Part print with two shaded views. Sizes in mm from the minimum x, y, z corner. A direction names the side the tool comes from. Give positions to 0.01 mm unless a question says otherwise; leave off trailing zeros. Loops run counter-clockwise (first coordinate to the right, second up) from the corner with the lowest first, then second, coordinate; pieces in that order, holes last. Notation, with made-up numbers: (-14, 10) -> (34, 10) arc R23 ccw to (34, 26) -> close; hole circle Ø10 at (36.5, 7). An arc over 180 degrees is marked (long way). One line per question, with ' | ' between items. Start each with the question number.
(1) Slice it at B-B, the plane x = 35.5. Write the cut outline in (y, z).
(2) Drill centre lines: L1, parallel to X at y = 7, z = 11.75; L2, parallel to Z at x = 14.5, y = 3. Where is each one in solid material? Low to high. Write a range as from..to.
(3) Mould opens along Z. For the marked faces 3, 4 and 5 say: pulls with the +Z half, pulls with the -Z half, needs draft (parallel to the pull), parting line crosses it, or undercut.
(4) 3-axis set-ups, long thin cutter, end or side, ignore diameter. For the marked faces 1 and 2: which of +Z, -Z, +X, -X, +Y, -Y reach the whole face in a straight line?
(5) Slice it at C-C, the plane z = 12.25. Write the cut outline in (x, y) (1 decimal).
(6) Slice it at A-A, the plane z = 19.25. Write the cut outline in (x, y).
(7) Flat gauge pins, fed straight in: pin 1 Ø9 at (y, z) = (12.37, 11.18) entering from +X; pin 2 Ø2 at (x, z) = (27.5, 17.5) entering from +Y. Where does each tip first touch, or does it go through?
(8) Slice it at D-D, the plane x = 3. Write the cut outline in (y, z) (1 decimal), then the cut area to 3 significant figures.
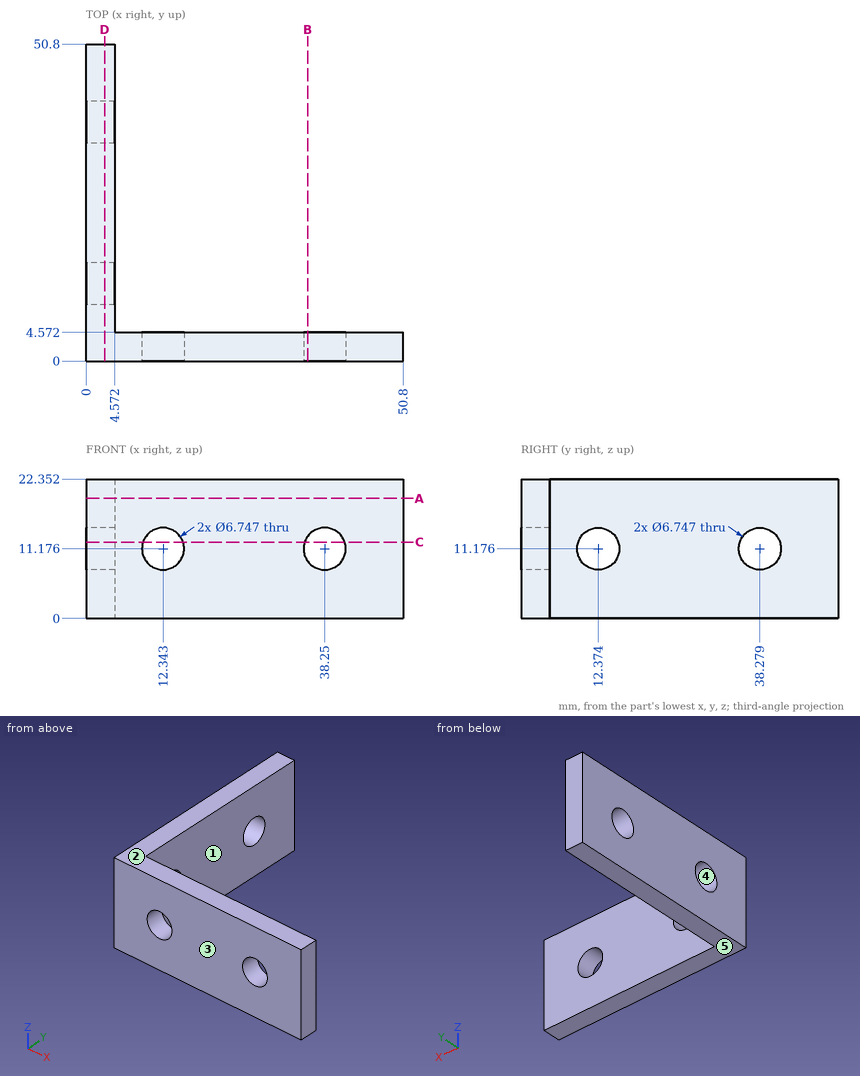
Final values:
1) outline: (0, 0) -> (4.57, 0) -> (4.57, 9.22) -> (0, 9.22) -> close; (0, 13.13) -> (4.57, 13.13) -> (4.57, 22.35) -> (0, 22.35) -> close
2) L1: 0..4.57 | L2: 0..8.58, 13.77..22.35
3) face 3: needs draft | face 4: undercut | face 5: pulls with the -Z half
4) face 1: +Z, -Z, +X, +Y | face 2: +Z, +X, -X, +Y, -Y
5) outline: (0, 0) -> (9.1, 0) -> (9.1, 4.6) -> (4.6, 4.6) -> (4.6, 9.2) -> (0, 9.2) -> close; (0, 15.6) -> (4.6, 15.6) -> (4.6, 35.1) -> (0, 35.1) -> close; (0, 41.5) -> (4.6, 41.5) -> (4.6, 50.8) -> (0, 50.8) -> close; (15.5, 0) -> (35.1, 0) -> (35.1, 4.6) -> (15.5, 4.6) -> close; (41.4, 0) -> (50.8, 0) -> (50.8, 4.6) -> (41.4, 4.6) -> close
6) outline: (0, 0) -> (50.8, 0) -> (50.8, 4.57) -> (4.57, 4.57) -> (4.57, 50.8) -> (0, 50.8) -> close
7) pin 1: x = 4.57 | pin 2: y = 4.57
8) outline: (0, 0) -> (50.8, 0) -> (50.8, 22.4) -> (0, 22.4) -> close; hole circle Ø6.7 at (12.4, 11.2); hole circle Ø6.7 at (38.3, 11.2) | area: 1,060 mm2
